Can you work these out from the model? Positions are in its coordinate system, mm. A direction names the side the tool comes from. Give positions to 0.01 mm unless a question says otherwise; leave off trailing zeros. Write each loop counter-clockwise with the first axis right and the second up, starting at its lowest first coordinate (ties: lowest second). Pieces come first, ordered by that corner, then holes. Notation, with made-up numbers: (48.5, 36) - (77.5, 36) arc R16 cw to (77.5, 52) - close; hole circle Ø11 at (33.25, 82). An arc over 180 degrees is marked (long way). Use a Markdown table: item, result. Add a question column.
```python
from build123d import *

# Parameters (mm, degrees)
F0_R     = 12.7
F1_DEPTH = 60.325
F3_DEPTH = 19.05
F4_W     = 32.8422
F4_H     = 41.275
F5_DEPTH = 34.798
F7_W     = 44.8917353029
F7_H     = 22.3266
F7_R     = 6.35
F8_DEPTH = 44.704
F9_R     = 3.302
F10_R    = 7.874
F11_R    = 5.08
F12_R    = 3.302


with BuildPart() as f1:
    # F0 (on Front) → F1 (new body)
    with BuildSketch(Plane.XZ):
        with BuildLine():
            ThreePointArc((-77.862515583, -22.352), (-62.0572648099, -15.8052507731), (-55.510515583, 0))
            ThreePointArc((-55.510515583, 0), (-93.6677663561, 15.8052507731), (-77.862515583, -22.352))
        make_face()
        with Locations((-77.862515583, 0)):
            Circle(F0_R, mode=Mode.SUBTRACT)
        with BuildLine():
            Line((39.383884417, 0), (-55.510515583, 0))
            ThreePointArc((-55.510515583, 0), (-62.0572648099, -15.8052507731), (-77.862515583, -22.352))
            Line((-77.862515583, -22.352), (116.345884417, -22.352))
            Line((116.345884417, -22.352), (116.345884417, 0))
            Line((116.345884417, 0), (72.226084417, 0))
            Line((72.226084417, 0), (72.226084417, 34.798))
            Line((72.226084417, 34.798), (53.176084417, 34.798))
            ThreePointArc((53.176084417, 34.798), (49.6018997785, 16.0823576341), (39.383884417, 0))
        make_face()
    extrude(amount=F1_DEPTH)

    # F2 (on face) → F3 (cut)
    with BuildSketch(Plane.XZ.offset(60.325)):
        Polygon((39.383884417, -22.352), (39.383884417, 0), (7.989484417, 0), (13.983884417, -22.352), align=None)
    extrude(amount=-F3_DEPTH, mode=Mode.SUBTRACT)

    # F4 (on face) → F5 (cut)
    with BuildSketch(Plane.XY.offset(34.798)):
        with Locations((55.804984417, -20.6375)):
            Rectangle(F4_W, F4_H)
    extrude(amount=-F5_DEPTH, mode=Mode.SUBTRACT)

    # F7 (on offset) → F8 (cut)
    with BuildSketch(Plane.XY.offset(22.352)):
        with Locations((-77.9563832345, -30.1625)):
            Rectangle(F7_W, F7_H)
        with Locations((77.483884417, -22.352)):
            Circle(F7_R)
    extrude(amount=-F8_DEPTH, mode=Mode.SUBTRACT)

    # F9
    f9_edges = [f1.edges().sort_by_distance(p)[0] for p in [
        (-55.510516, -50.8254, 0),
        (-55.510516, -9.4996, 0),
    ]]
    fillet(f9_edges, radius=F9_R)

    # F10
    f10_edges = [f1.edges().sort_by_distance(p)[0] for p in [
        (116.345884, -30.1625, 0),
    ]]
    fillet(f10_edges, radius=F10_R)

    # F11
    f11_edges = [f1.edges().sort_by_distance(p)[0] for p in [
        (72.226084, -50.8, 34.798),
    ]]
    fillet(f11_edges, radius=F11_R)

    # F12
    f12_edges = [f1.edges().sort_by_distance(p)[0] for p in [
        (72.226084, -50.8, 0),
    ]]
    fillet(f12_edges, radius=F12_R)


solid = f1.part
```
Q1. I'm going to push flat-ended pins straight in: P1, Ø2, axis at y = -7, z = 4, coming from the -X side; P2, Ø2, axis at x = 49.5, z = -5, coming from the +Y side; P3, Ø8, axis at y = -11, z = 24, coming from the -X side; P4, Ø5, axis at y = -45, z = 19, coming from the -X side. Where does each tip first touch, or does it pass through?
Q2. On a 3-axis mill with a long thin cutter (end or side, diameter ignored), from which of +Z, -Z, +X, -X, +Y, -Y can I reach the whole of each face in a straight line? I mean faces 5 (the flat face through (39.384, -51, -11)), 6 (the flat face through (10.945, -50.933, -11.02)), 7 (the flat face through (72.226, -51, 16)), 8 (the flat face through (116.346, -30, -15)). Say none if no direction works.
Q3. If we mould it in two halves opening along Y, with no side actions, what happens to faces 1 (the flat face through (-66, -18.999, -5)), 2 (the cylindrical face through (-66.13, -50.69, -4.86)), 3 (the flat face through (23, -41.275, -11)), 4 (the flat face through (-55.511, -30, -11))? For each: released by +Y, released by -Y, zero draft, split by the parting line, or undercut.
Q4. Suppose I cut it at C-C (x = -31). Please give me the cut outline in (y, z) (3 decimals), and give its area (3 significant figures).
Q5. Suppose I cut it at D-D (x = 16). Please give me the cut outline in (y, z) (3 decimals).
Q6. If I drill on probe 1 along Z at (x, y) = (1, -40); probe 2 along Z at (x, y) = (-87, -13.5); probe 3 along Y at (x, z) = (12, -6.5) (3 decimals), over which ranges is the centre line in solid material (lowest first)? Write a range as [from, to].
Q7. Suppose I cut it at B-B (x = 65). Please give me the cut outline in (y, z) (3 decimals), and give its area (3 significant figures).
Q8. Suppose I cut it at A-A (y = -55). Please give me the cut outline in (x, z).
Derived:
| question | item | result |
|---|---|---|
| 1 | P1 | x = -100.01 |
| 1 | P2 | y = 0 |
| 1 | P3 | x = -87.84 |
| 1 | P4 | x = -92.94 |
| 2 | face 5 | +Z, -Z, -Y |
| 2 | face 6 | +Z, -Y |
| 2 | face 7 | +Z, +X, +Y, -Y |
| 2 | face 8 | +Z, -Z, +X, +Y, -Y |
| 3 | face 1 | undercut |
| 3 | face 2 | zero draft |
| 3 | face 3 | released by -Y |
| 3 | face 4 | undercut |
| 4 | outline | (-60.325, -22.352) - (0, -22.352) - (0, 0) - (-60.325, 0) - close |
| 4 | area | 1,350 mm² |
| 5 | outline | (-41.275, -22.352) - (0, -22.352) - (0, 0) - (-41.275, 0) - close |
| 6 | probe 1 | [-22.35, 0] |
| 6 | probe 2 | [-20.4, -8.82], [8.82, 20.4] |
| 6 | probe 3 | [-41.275, 0] |
| 7 | outline | (-60.325, -22.352) - (0, -22.352) - (0, 0) - (-41.275, 0) - (-41.275, 34.798) - (-60.325, 34.798) - close |
| 7 | area | 2,010 mm² |
| 8 | outline | (-77.86, -22.35) - (13.98, -22.35) - (7.99, 0) - (-52.42, 0) arc R3.3 cw to (-55.7, 2.88) arc R22.35 ccw (long way) to start; (39.38, -22.35) - (116.35, -22.35) - (116.35, -7.87) arc R7.87 ccw to (108.47, 0) - (75.53, 0) arc R3.3 cw to (72.23, 3.3) - (72.23, 29.72) arc R5.08 ccw to (67.15, 34.8) - (53.18, 34.8) arc R50.8 cw to (39.38, 0) - close; hole circle Ø25.4 at (-77.86, 0) |
